Can you work these out from the model? Positions are in its coordinate system, mm. A direction names the side the tool comes from. Coordinates: 2 decimals unless noted, no trailing zeros. Order: outer loops, then holes, each group sorted by start corner. A loop starts at its lowest first (then second) coordinate and runs counter-clockwise, first axis right, second up. Notation, with made-up numbers: M 68,33 L 121,33 A20 ccw 121,72 Z; hole C 33,79.25 d1. An arc over 180 degrees is marked long. Answer as a JSON object with one key per item and string values.
from build123d import *

# Parameters (mm, degrees)
F1_DEPTH = 75
F4_DEPTH = 200
F5_DEPTH = 100


# Not quite as in the source:
# - ends of sketch curves that miss each other by under 0.0002 mm in the source are joined


with BuildPart() as f1:
    # F0 (on Front) → F1 (new body, symmetric)
    with BuildSketch(Plane.XZ):
        Polygon((64.9607930725, 65.0385569036), (-20.0392069275, 65.0385569036), (-105.0392069275, 65.0385569036), (-105.0392069275, 35.0244045258), (-29.7518869333, 10.1945746155), (-20.0392069275, 39.6446734667), (-10.3405706844, 10.2371571158), (64.9607930725, 35.0385569036), align=None)
    extrude(amount=F1_DEPTH, both=True)

    # F2 (on face) → F4 (cut)
    with BuildSketch(Plane.XZ.offset(75)):
        Polygon((-100.0392069275, 38.640326764), (-32.9342746626, 16.5090348727), (-20.0392069275, 55.6085438923), (-7.1575624177, 16.5497358238), (59.9607930725, 38.6559645103), (59.9607930725, 60.0385569036), (-100.0392069275, 60.0385569036), align=None)
    extrude(amount=-F4_DEPTH, mode=Mode.SUBTRACT)

    # F3 (on face) → F5 (intersect)
    with BuildSketch(Plane.XY.offset(65.0385569036)):
        with BuildLine():
            Line((-107.177117556, 42.4698600353), (-115.9930899739, 40.6591594219))
            ThreePointArc((-115.9930899739, 40.6591594219), (-18.9798846841, -38.4537255363), (78.0333206058, 40.6591594219))
            Line((78.0333206058, 40.6591594219), (69.2173481878, 42.4698600353))
            ThreePointArc((69.2173481878, 42.4698600353), (-18.9798846841, -29.4537251816), (-107.177117556, 42.4698600353))
        make_face()
    extrude(amount=-F5_DEPTH, mode=Mode.INTERSECT)


solid = f1.part
Item 1: Please list where these lines run through material, in increasing order: line 1 (X direction, y = 5.5, z = 59); line 2 (Z direction, x = 17, y = -22); line 3 (X direction, y = 6, z = 39).
Answers follow:
{"line 1": "x = -101.29 to -100.04, 59.96 to 63.33", "line 2": "z = 19.24 to 24.51, 60.04 to 65.04", "line 3": "x = -101.62 to -100.04, 59.96 to 63.66"}
Item 2: Which directions (+Z, -Z, +X, -X, +Y, -Y) give clear straight access to the entire face, cutting with the end or side of a thin tool? Please do faces 1 (the flat face through (-26.577, -33.478, 35.785)), 2 (the flat face through (32.712, -14.977, 24.417)).
Answers follow:
{"face 1": "+Y, -Y", "face 2": "-Z, +X, +Y, -Y"}
Item 3: If we mould it in two halves opening along X, with no side actions, what happens to faces 3 (the flat face through (-26, -32, 65.039)), 4 (the flat face through (-73.148, -12.708, 24.507)), 5 (the flat face through (64.961, 18, 50)), 6 (the flat face through (28.73, -16.48, 28.37))? For each: pulls with the +X half, pulls with the -X half, needs draft (parallel to the pull), parting line crosses it, or undercut.
Answers follow:
{"face 3": "needs draft", "face 4": "pulls with the -X half", "face 5": "pulls with the +X half", "face 6": "undercut"}
Item 4: I'm going to push flat-ended pins straight in: pin 1 (12 mm diameter, centred on x = -45, z = 31, fed in from -Y); pin 2 (4 mm diameter, centred on y = 0.5, z = 48.5, fed in from +X); pin 3 (13 mm diameter, centred on y = 9, z = 48.5, fed in from -X); pin 4 (6 mm diameter, centred on y = -24.5, z = 23, fed in from +X). Where does each tip first touch, or does it pass through?
Answers follow:
{"pin 1": "passes through", "pin 2": "stops at x = 61.24", "pin 3": "stops at x = -105.04", "pin 4": "stops at x = 35.02"}
Item 5: I want a section at C-C, the plane z = 26. Write out the boundary of the cut face in (x, y), plus the area to 3 significant figures.
Answers follow:
{"outline": "M -77.68,-19.19 A99.04 ccw -61.71,-28.76 L -61.71,-18.67 A90.04 cw -77.68,-7.69 Z; M -29.8,-37.86 A99.04 ccw -24.54,-38.3 L -24.54,-29.28 A90.04 cw -29.8,-28.8 Z; M -15.54,-38.39 A99.04 ccw -10.27,-38.07 L -10.27,-29.03 A90.04 cw -15.54,-29.39 Z; M 21.54,-29.79 A99.04 ccw 37.52,-20.76 L 37.52,-9.52 A90.04 cw 21.54,-19.82 Z", "area": "434 mm^2"}
Item 6: I want a section at D-D, the plane x = -27.5. Write out the boundary of the cut face in (y, z).
Answers follow:
{"outline": "M -38.09,17.02 L -29.05,17.02 L -29.05,32.99 L -38.09,32.99 Z; M -38.09,60.04 L -29.05,60.04 L -29.05,65.04 L -38.09,65.04 Z"}
Item 7: I want a section at A-A, the plane z = 58. Write out the boundary of the cut face in (x, y).
Answers follow:
{"outline": "M -105.04,11.57 A99.04 ccw -100.04,3.68 L -100.04,21.39 A90.04 cw -105.04,34.11 Z; M 59.96,0.78 A99.04 ccw 64.96,8.02 L 64.96,28.01 A90.04 cw 59.96,17.28 Z"}
Item 8: I want a section at B-B, the plane y = 13.5. Write out the boundary of the cut face in (x, z), plus the area to 3 significant figures.
Answers follow:
{"outline": "M -105.04,35.02 L -95.73,31.95 L -95.73,37.22 L -100.04,38.64 L -100.04,60.04 L -95.73,60.04 L -95.73,65.04 L -105.04,65.04 Z; M 57.77,32.67 L 64.96,35.04 L 64.96,65.04 L 57.77,65.04 L 57.77,60.04 L 59.96,60.04 L 59.96,38.66 L 57.77,37.93 Z", "area": "375 mm^2"}
